Check sheet for the modelled part. Datum: model origin and axes. Units: mm. A direction names the side the tool comes from. Coordinates: 2 decimals unless noted, no trailing zeros. Loops run counter-clockwise (first coordinate to the right, second up) from the corner with the lowest first, then second, coordinate; pieces in that order, holes last. Notation, with made-up numbers: (-15, 72.25) -> (2, 72.25) arc R28 cw to (2, 108.25) -> close; hole circle Ø9 at (12, 82.5). An arc over 180 degrees is marked (long way). Use CSV: the item, a comma, the result in double quotes.
```python
from build123d import *

# Parameters (mm, degrees)
EXTRUDE1_DEPTH = 3
EXTRUDE2_DEPTH = 66
EXTRUDE3_START = -3
EXTRUDE3_DEPTH = 3
SKETCH2_R      = 2
EXTRUDE4_DEPTH = 3
EXTRUDE5_START = -3
SKETCH6_R      = 2
EXTRUDE5_DEPTH = 3
FILLET3_R      = 3.5
FILLET6_R      = 2
FILLET7_R      = 0.5
FILLET13_R     = 2


with BuildPart() as part:
    # Sketch1 → Extrude1 (new body)
    with BuildSketch(Plane.XY):
        with BuildLine():
            Line((-14.803266257, -5.201299994), (-2.663266257, 6.938700006))
            Line((-2.663266257, 6.938700006), (-2.663266257, 8.94083563))
            ThreePointArc((-2.663266257, 8.94083563), (3.336733743, 14.94083563), (9.336733743, 8.94083563))
            Line((9.336733743, 8.94083563), (9.336733743, 4.94083563))
            Line((9.336733743, 4.94083563), (-10.803266257, -9.201299994))
            Line((-10.803266257, -9.201299994), (-10.803266257, -5.201299994))
            Line((-10.803266257, -5.201299994), (-14.803266257, -5.201299994))
        make_face()
    extrude(amount=EXTRUDE1_DEPTH)

    # Sketch3 → Extrude2 (add)
    with BuildSketch(Plane.XY):
        Polygon((-14.803266257, -5.201299994), (-10.803266257, -5.201299994), (-10.803266257, -13.596193084), (-23.198159347, -13.596193084), align=None)
    extrude(amount=EXTRUDE2_DEPTH)

    # Sketch4 → Extrude3 (add)
    with BuildSketch(Plane.XY.offset(66).offset(EXTRUDE3_START)):
        with BuildLine():
            Line((-14.803266257, -5.201299994), (-10.803266257, -5.201299994))
            Line((-10.803266257, -5.201299994), (-10.803266257, -9.201299994))
            Line((-10.803266257, -9.201299994), (9.336733743, 4.94083563))
            Line((9.336733743, 4.94083563), (9.336733743, 8.94083563))
            ThreePointArc((9.336733743, 8.94083563), (3.336733743, 14.94083563), (-2.663266257, 8.94083563))
            Line((-2.663266257, 8.94083563), (-2.663266257, 6.938700006))
            Line((-2.663266257, 6.938700006), (-14.803266257, -5.201299994))
        make_face()
    extrude(amount=EXTRUDE3_DEPTH)

    # Sketch2 → Extrude4 (cut)
    with BuildSketch(Plane.XY.offset(3)):
        with Locations((3.336733743, 8.94083563)):
            Circle(SKETCH2_R)
    extrude(amount=-EXTRUDE4_DEPTH, mode=Mode.SUBTRACT)

    # Sketch6 → Extrude5 (cut)
    with BuildSketch(Plane(origin=(0, 0, 63), x_dir=(-1, 0, 0), z_dir=(0, 0, -1)).offset(EXTRUDE5_START)):
        with Locations(Location((-3.336733743, 8.94083563, 0), (0, 0, 180))):
            Circle(SKETCH6_R)
    extrude(amount=EXTRUDE5_DEPTH, mode=Mode.SUBTRACT)

    # Fillet3
    fillet3_edges = [part.edges().sort_by_distance(p)[0] for p in [
        (-12.803266257, -5.201299994, 3),
        (-12.803266257, -5.201299994, 63),
    ]]
    fillet(fillet3_edges, radius=FILLET3_R)

    # Fillet6
    fillet6_edges = [part.edges().sort_by_distance(p)[0] for p in [
        (9.336733743, 4.94083563, 1.5),
        (-2.663266257, 6.938700006, 1.5),
        (-2.663266257, 6.938700006, 64.5),
        (9.336733743, 4.94083563, 64.5),
    ]]
    fillet(fillet6_edges, radius=FILLET6_R)

    # Fillet7
    fillet7_edges = [part.edges().sort_by_distance(p)[0] for p in [
        (-23.198159347, -13.596193084, 33),
    ]]
    fillet(fillet7_edges, radius=FILLET7_R)

    # Fillet13
    fillet13_edges = [part.edges().sort_by_distance(p)[0] for p in [
        (-10.803266257, -9.201299994, 1.5),
        (-10.803266257, -13.596193084, 33),
        (-10.803266257, -9.201299994, 64.5),
    ]]
    fillet(fillet13_edges, radius=FILLET13_R)


solid = part.part
```
1) Go/stop test with flat-tipped pins: pin 1 Ø5 at (y, z) = (-4.5, 34.5) entering from +X; pin 2 Ø3 at (x, y) = (-2.5, -5.5) entering from -Z; pin 3 Ø8 at (y, z) = (-7.5, 56.5) entering from -X; pin 4 Ø4.5 at (x, z) = (-13, 31) entering from +Y. Record where each tip stops, or that it passes through.
Answer below:
pin 1,"stops at x = -10.8"
pin 2,"passes through"
pin 3,"stops at x = -21.1"
pin 4,"stops at y = -5.2"
2) Cross-section at D-D on z = 48.5. Record the boundary of the cut face in (x, y), and give its area (3 significant figures).
Answer below:
outline,"(-22.34, -12.74) arc R0.5 ccw to (-21.99, -13.6) -> (-12.8, -13.6) arc R2 ccw to (-10.8, -11.6) -> (-10.8, -5.2) -> (-14.8, -5.2) -> close"
area,"67.6 mm²"
3) Draft check along Z on faces 1 (the flat face through (-4, 0, 0)), 2 (the flat face through (-1, 3, 63)), 3 (the cylindrical face through (-2.82, 6.99, 64.52)). Enter one of: released by +Z, released by -Z, zero draft, split by the parting line, or undercut.
Answer below:
face 1,"released by -Z"
face 2,"undercut"
face 3,"zero draft"
4) Cross-section at B-B on y = -1. Record the boundary of the cut face in (x, z), and give its area (3 significant figures).
Answer below:
outline,"(-10.6, 0) -> (0.88, 0) -> (0.88, 3) -> (-10.6, 3) -> close; (-10.6, 63) -> (0.88, 63) -> (0.88, 66) -> (-10.6, 66) -> close"
area,"68.9 mm²"
5) Cross-section at C-C on x = -4. Record the boundary of the cut face in (y, z).
Answer below:
outline,"(-4.42, 0) -> (5.6, 0) -> (5.6, 3) -> (-4.42, 3) -> close; (-4.42, 63) -> (5.6, 63) -> (5.6, 66) -> (-4.42, 66) -> close"
6) Access from +Z, -Z, +X, -X, +Y, -Y to the whole of each face (thin tool, end or side, straight path). Record for faces 4 (the cylindrical face through (3.47, 14.94, 64.48)), 5 (the flat face through (-13, -5.201, 33)).
Answer below:
face 4,"+Z, -Z, +Y"
face 5,"+X, -X, +Y"
7) Thickness scan on line 1 along Z through (x, y) = (2.5, 11); line 2 along Y through (x, z) = (-14.5, 39); line 3 along Y through (x, z) = (-16, 10). Record the ranges inside material, lowest first. Write a range as from..to.
Answer below:
line 1,"z = 0..3, 63..66"
line 2,"y = -13.6..-5.2"
line 3,"y = -13.6..-6.4"
8) Cross-section at A-A on x = 4. Record the boundary of the cut face in (y, z), and give its area (3 significant figures).
Answer below:
outline,"(1.19, 0) -> (7.05, 0) -> (7.05, 3) -> (1.19, 3) -> close; (1.19, 63) -> (7.05, 63) -> (7.05, 66) -> (1.19, 66) -> close; (10.83, 0) -> (14.9, 0) -> (14.9, 3) -> (10.83, 3) -> close; (10.83, 63) -> (14.9, 63) -> (14.9, 66) -> (10.83, 66) -> close"
area,"59.6 mm²"
